Design review of the part built by this model. Coordinates are the model's own, in mm. Coordinates: 2 decimals unless noted, no trailing zeros. Write each loop counter-clockwise with the first axis right and the second up, starting at its lowest first coordinate (ties: lowest second). Pieces come first, ordered by that corner, then holes.
Q1. For pin 1 Ø7.5 at (x, z) = (2.5, 6.5) entering from +Y; pin 2 Ø2 at (x, y) = (-5, 7) entering from -Z; pin 3 Ø6 at (y, z) = (24, -11) entering from -X; pin 4 Ø12 at (y, z) = (2, -12) entering from -X, all flat-tipped, find the tip position at first contact; note any pin that passes through.
Q2. For L1, parallel to Y at x = 2.5, z = -21; L2, parallel to X at y = 27.5, z = -4.5; L3, parallel to X at y = 17, z = 0, list the stretches that pass through material, from the lowest coordinate up.
Q3. Take a section at B-B, the plane y = 13.5. Write out the cut boundary in (x, z).
Q4. The part is to be moulded in two halves that separate along Z. For faces 1 (the flat face through (2.966, -5.087, -32.075)), 2 (the flat face through (0, 7.938, -3)), 3 (the flat face through (1.02, 19.05, -2.23)), 4 (the flat face through (-6.84, -5.09, 11.59)), say which applies: released by +Z, released by -Z, zero draft, split by the parting line, or undercut.
Q5. Take a section at C-C, the plane z = -27. Write out the cut boundary in (x, y), plus the area to 3 significant figures.
from build123d import *

# Parameters (mm, degrees)
F4_DEPTH = 10.31875
F1_R     = 6.746875
F5_DEPTH = 30.48
F6_DEPTH = 35.3822
F7_DEPTH = 7.9375


with BuildPart() as f4:
    # F0 (on Front) → F4 (new body)
    with BuildSketch(Plane.XZ):
        with BuildLine():
            Line((-7.342188, 5.953125), (-7.14375, 0))
            Line((-7.14375, 0), (7.14375, 0))
            Line((7.14375, 0), (7.342187, 5.953125))
            Line((7.342187, 5.953125), (6.35, 17.065625))
            Line((6.35, 17.065625), (4.13357, 25.340298))
            ThreePointArc((4.13357, 25.340298), (2.602599, 27.338054), (0.23001, 28.178125))
            Line((0.23001, 28.178125), (-0.23001, 28.178125))
            ThreePointArc((-0.23001, 28.178125), (-2.602599, 27.338054), (-4.13357, 25.340298))
            Line((-4.13357, 25.340298), (-6.35, 17.065625))
            Line((-6.35, 17.065625), (-7.342188, 5.953125))
        make_face()
        with BuildLine():
            Line((7.14375, 0), (-7.14375, 0))
            Line((-7.14375, 0), (-6.35, -11.1125))
            Line((-6.35, -11.1125), (-5.55625, -20.6375))
            Line((-5.55625, -20.6375), (-4.365625, -28.575))
            Line((-4.365625, -28.575), (-1.63132, -35.410762))
            ThreePointArc((-1.63132, -35.410762), (-1.007245, -36.195929), (-0.055542, -36.5125))
            Line((-0.055542, -36.5125), (0.057313, -36.5125))
            ThreePointArc((0.057313, -36.5125), (0.979065, -36.216412), (1.604621, -35.477511))
            Line((1.604621, -35.477511), (4.365625, -28.575))
            Line((4.365625, -28.575), (5.55625, -20.6375))
            Line((5.55625, -20.6375), (6.35, -11.1125))
            Line((6.35, -11.1125), (7.14375, 0))
        make_face()
        with BuildLine():
            ThreePointArc((0.23001, 28.178125), (0, 28.184106), (-0.23001, 28.178125))
            Line((-0.23001, 28.178125), (0.23001, 28.178125))
        make_face()
        with BuildLine():
            Line((0.057313, -36.5125), (-0.055542, -36.5125))
            ThreePointArc((-0.055542, -36.5125), (0.000885, -36.513405), (0.057313, -36.5125))
        make_face()
    extrude(amount=F4_DEPTH)

    # F1 (on Front) → F5 (join)
    with BuildSketch(Plane.XZ):
        with Locations((0, -3.175531)):
            Circle(F1_R)
    extrude(amount=-F5_DEPTH)

    # F2 (on Front) → F6 (cut)
    with BuildSketch(Plane.XZ):
        Polygon((-1.543482, 0.332913), (-2.525697, -0.649303), (-3.507913, -1.631518), (1.543482, -6.682913), (2.525697, -5.700697), (3.507913, -4.718482), align=None)
    extrude(amount=-F6_DEPTH, mode=Mode.SUBTRACT)

    # F3 (on Front) → F7 (join)
    with BuildSketch(Plane.XZ):
        Polygon((-1.543482, 0.332913), (-2.525697, -0.649303), (-3.507913, -1.631518), (1.543482, -6.682913), (2.525697, -5.700697), (3.507913, -4.718482), align=None)
    extrude(amount=-F7_DEPTH)


solid = f4.part
Responses:
1. pin 1: stops at y = 30.48
1. pin 2: stops at z = -8.61
1. pin 3: stops at x = -4.72
1. pin 4: stops at x = -6.69
2. L1: y = -10.32 to 0
2. L2: x = -6.62 to -0.64, 3.29 to 6.62
2. L3: x = -5.95 to -1.88, -1.21 to 5.95
3. outline: circle Ø13.49 at (0, -3.18); hole (-3.51, -1.63) - (1.54, -6.68) - (2.53, -5.7) - (3.51, -4.72) - (-1.54, 0.33) - (-2.53, -0.65) - close
4. face 1: released by -Z
4. face 2: undercut
4. face 3: undercut
4. face 4: released by +Z
5. outline: (-4.6, -10.32) - (4.6, -10.32) - (4.6, 0) - (-4.6, 0) - close
5. area: 95.0 mm2
